```python
from build123d import *

# Parameters (mm, degrees)
SKETCH2_W                   = 177.8
SKETCH2_H                   = 152.4
BOSS_EXTRUDE1_DEPTH         = 6.35
F_3_8_CLEARANCE_HOLE1_D     = 10.0838
TAP_DRILL_FOR_1_4_20_TAP1_D = 5.1054
TAP_DRILL_FOR_3_8_16_TAP3_D = 7.9375
F_1_4_0_25_DIAMETER_HOLE1_D = 6.35
CUT_EXTRUDE2_DEPTH          = 235.26250767
CUT_EXTRUDE3_DEPTH          = 235.26250767


with BuildPart() as part:
    # Sketch2 → Boss-Extrude1 (new body)
    with BuildSketch(Plane(origin=(0, 0, 0), x_dir=(0, 1, 0), z_dir=(0, 0, 1))):
        with Locations((88.9, 76.2)):
            Rectangle(SKETCH2_W, SKETCH2_H)
    extrude(amount=BOSS_EXTRUDE1_DEPTH)

    # 3/8 Clearance Hole1 (through all)
    with Locations(Plane.XY.offset(6.35)):
        with Locations((-101.6, 63.5), (-139.7, 63.5), (-139.7, 165.1)):
            Hole(F_3_8_CLEARANCE_HOLE1_D / 2)

    # Tap Drill for 1/4-20 Tap1 (through all)
    with Locations(Plane.XY.offset(6.35)):
        with Locations((-27.75458, 84.8487), (-36.24072, 122.02414)):
            Hole(TAP_DRILL_FOR_1_4_20_TAP1_D / 2)

    # Tap Drill for 3/8-16 Tap3 (through all)
    with Locations(Plane(origin=(0, 0, 0), x_dir=(1, 0, 0), z_dir=(0, 0, -1))):
        with Locations((-58.656709878, -161.952743754), (-19.260612718, -39.85289442)):
            Hole(TAP_DRILL_FOR_3_8_16_TAP3_D / 2)

    # 1/4 (0.25) Diameter Hole1 (through all)
    with Locations(Plane(origin=(0, 0, 0), x_dir=(1, 0, 0), z_dir=(0, 0, -1))):
        with Locations((-101.6, -88.9), (-139.7, -139.7)):
            Hole(F_1_4_0_25_DIAMETER_HOLE1_D / 2)

    # Sketch22 → Cut-Extrude2 (cut, through all)
    with BuildSketch(Plane(origin=(0, 0, 0), x_dir=(1, 0, 0), z_dir=(0, 0, -1))):
        with BuildLine():
            Line((-29.480310158, -143.097334182), (-33.290310158, -136.498220605))
            ThreePointArc((-33.290310158, -136.498220605), (-32.692975, -134.268935448), (-30.463689842, -134.866270605))
            Line((-30.463689842, -134.866270605), (-26.653689842, -141.465384182))
            ThreePointArc((-26.653689842, -141.465384182), (-27.251025, -143.69466934), (-29.480310158, -143.097334182))
        make_face()
        with BuildLine():
            Line((-29.480310158, -169.933729395), (-41.037310158, -149.916418212))
            ThreePointArc((-41.037310158, -149.916418212), (-40.439975, -147.687133054), (-38.210689842, -148.284468212))
            Line((-38.210689842, -148.284468212), (-26.653689842, -168.301779395))
            ThreePointArc((-26.653689842, -168.301779395), (-27.251025, -170.531064552), (-29.480310158, -169.933729395))
        make_face()
        with BuildLine():
            Line((-13.986310158, -169.933729395), (-17.796310158, -163.334615818))
            ThreePointArc((-17.796310158, -163.334615818), (-17.198975, -161.10533066), (-14.969689842, -161.702665818))
            Line((-14.969689842, -161.702665818), (-11.159689842, -168.301779395))
            ThreePointArc((-11.159689842, -168.301779395), (-11.757025, -170.531064552), (-13.986310158, -169.933729395))
        make_face()
    extrude(amount=-CUT_EXTRUDE2_DEPTH, mode=Mode.SUBTRACT)

    # Sketch20 → Cut-Extrude3 (cut, through all)
    with BuildSketch(Plane(origin=(0, 0, 0), x_dir=(1, 0, 0), z_dir=(0, 0, -1))):
        with BuildLine():
            Line((-19.385125577, -155.159806788), (-23.195125577, -148.560693212))
            ThreePointArc((-23.195125577, -148.560693212), (-20.987077328, -140.320144963), (-12.74652908, -142.528193212))
            Line((-12.74652908, -142.528193212), (-8.93652908, -149.127306788))
            ThreePointArc((-8.93652908, -149.127306788), (-11.144577328, -157.367855037), (-19.385125577, -155.159806788))
        make_face()
    extrude(amount=-CUT_EXTRUDE3_DEPTH, mode=Mode.SUBTRACT)


solid = part.part
```
Work out the finished part from the listing and answer in its coordinate system (mm). A direction names the side the tool comes from. Round coordinates to 2 decimals unless told otherwise and drop trailing zeros. Write each loop counter-clockwise with the first axis right and the second up, starting at its lowest first coordinate (ties: lowest second). Pieces come first, ordered by that corner, then holes. Notation, with made-up numbers: (64.5, 16) - (93.5, 16) arc R7 cw to (93.5, 29) - close; hole circle Ø3 at (-21, 27). An arc over 180 degrees is marked (long way). Return JSON: item names as keys, results as strings. Group by question number.
Q1. The mould has two halves that part along Y. Classify faces 3 (the flat face through (-28.585, 138.12, 3.131)), 4 (the flat face through (-75, 0, 3)), 5 (the flat face through (-77, 88, 0)): released by +Y, released by -Y, zero draft, split by the parting line, or undercut.
Q2. The part is cut by section C-C on x = -139.7. Write down the section's boundary in (y, z) (3 decimals), then the cut area to 3 significant figures.
Q3. The part is cut by section D-D on z = 2.25. Count the separate pieces of the cut face and the enclosed holes in it, then the cut area to 3 significant figures.
Q4. Each of these flat-tipped pins is pushed along its axis until it touches: pin 1 Ø16 at (x, y) = (-101.6, 63.5) entering from -Z; pin 2 Ø5.5 at (x, y) = (-101.6, 88.9) entering from +Z. Where does it stop, or does it pass through?
Q5. Find the intervals of material crossed by L1, parallel to Y at x = -101.6, z = 3.75 (3 decimals); L2, parallel to Y at x = -35, z = 3.25; L3, parallel to X at y = 152.5, z = 2, in increasing order.
Q6. The part is cut by section B-B on y = 63.5. Write down the section's boundary in (x, z).
Q7. The part is cut by section A-A on x = -101.6. Write down the section's boundary in (y, z) (3 decimals), then the cut area to 3 significant figures.
Q8. For faces 1 (the flat face through (-152.4, 88, 3)), 2 (the flat face through (-31.36, 139.84, 3.13)), determine the directions among +Z, -Z, +X, -X, +Y, -Y from which every point of the face is accessible in a straight line to the end or side of a thin tool.
Solved:
{
 "1": {"face 3": "undercut", "face 4": "released by -Y", "face 5": "zero draft"},
 "2": {"outline": "(0, 0) - (58.458, 0) - (58.458, 6.35) - (0, 6.35) - close; (68.542, 0) - (136.525, 0) - (136.525, 6.35) - (68.542, 6.35) - close; (142.875, 0) - (160.058, 0) - (160.058, 6.35) - (142.875, 6.35) - close; (170.142, 0) - (177.8, 0) - (177.8, 6.35) - (170.142, 6.35) - close", "area": "961 mm²"},
 "3": {"separate pieces": "1", "enclosed holes": "13", "area": "26,300 mm²"},
 "4": {"pin 1": "z = 0", "pin 2": "through"},
 "5": {"L1": "0 to 58.458, 68.542 to 85.725, 92.075 to 177.8", "L2": "0 to 119.79, 124.26 to 153.85, 160.37 to 177.8", "L3": "-152.4 to -39.55, -35.78 to -20.92, -8.14 to 0"},
 "6": {"outline": "(-152.4, 0) - (-144.74, 0) - (-144.74, 6.35) - (-152.4, 6.35) - close; (-134.66, 0) - (-106.64, 0) - (-106.64, 6.35) - (-134.66, 6.35) - close; (-96.56, 0) - (0, 0) - (0, 6.35) - (-96.56, 6.35) - close"},
 "7": {"outline": "(0, 0) - (58.458, 0) - (58.458, 6.35) - (0, 6.35) - close; (68.542, 0) - (85.725, 0) - (85.725, 6.35) - (68.542, 6.35) - close; (92.075, 0) - (177.8, 0) - (177.8, 6.35) - (92.075, 6.35) - close", "area": "1,020 mm²"},
 "8": {"face 1": "+Z, -Z, -X, +Y, -Y", "face 2": "+Z, -Z"}
}
